Work out the finished part from the listing and answer in its coordinate system (mm). A direction names the side the tool comes from. Coordinates: 2 decimals unless noted, no trailing zeros. Loops run counter-clockwise (first coordinate to the right, second up) from the corner with the lowest first, then second, coordinate; pieces in that order, holes last.
```python
from build123d import *

# Parameters (mm, degrees)
SKETCH_1_W          = 109
SKETCH_1_H          = 63
EXTRUDE_1_DEPTH     = 5
CHAMFER_1_SIZE      = 3
SKETCH_2_W          = 75
SKETCH_2_H          = 45
EXTRUDE_2_DEPTH     = 20
SKETCH_3_W          = 70
SKETCH_3_H          = 27
CUT_EXTRUDE_1_DEPTH = 18
SKETCH_4_W          = 73
SKETCH_4_H          = 43
CUT_EXTRUDE_2_DEPTH = 15
SKETCH_5_R          = 2
EXTRUDE_3_DEPTH     = 10
FILLET_1_R          = 2


with BuildPart() as part:
    # 草图1 → 凸台-拉伸1 (new body)
    with BuildSketch(Plane.XY):
        Rectangle(SKETCH_1_W, SKETCH_1_H)
    extrude(amount=EXTRUDE_1_DEPTH)

    # 倒角1
    chamfer_1_edges = [part.edges().sort_by_distance(p)[0] for p in [
        (-54.5, 0, 5),
        (0, -31.5, 5),
        (54.5, 0, 5),
        (0, 31.5, 5),
    ]]
    chamfer(chamfer_1_edges, length=CHAMFER_1_SIZE)

    # 草图2 → 凸台-拉伸2 (add)
    with BuildSketch(Plane.XY.offset(5)):
        Rectangle(SKETCH_2_W, SKETCH_2_H)
    extrude(amount=-EXTRUDE_2_DEPTH)

    # 草图3 → 切除-拉伸1 (cut)
    with BuildSketch(Plane.XY.offset(5)):
        Rectangle(SKETCH_3_W, SKETCH_3_H)
    extrude(amount=-CUT_EXTRUDE_1_DEPTH, mode=Mode.SUBTRACT)

    # 草图4 → 切除-拉伸2 (cut)
    with BuildSketch(Plane.XY.offset(-13)):
        Rectangle(SKETCH_4_W, SKETCH_4_H)
    extrude(amount=CUT_EXTRUDE_2_DEPTH, mode=Mode.SUBTRACT)

    # 草图5 → 凸台-拉伸3 (add)
    with BuildSketch(Plane(origin=(0, 0, 0), x_dir=(-1, 0, 0), z_dir=(0, 0, -1))):
        with Locations((44, 19)):
            Circle(SKETCH_5_R)
        with Locations((44, -19)):
            Circle(SKETCH_5_R)
        with Locations((-44, -19)):
            Circle(SKETCH_5_R)
        with Locations((-44, 19)):
            Circle(SKETCH_5_R)
    extrude(amount=EXTRUDE_3_DEPTH)

    # 圆角1
    fillet_1_edges = [part.edges().sort_by_distance(p)[0] for p in [
        (37.5, 0, -15),
        (0, -22.5, -15),
        (-37.5, 0, -15),
        (0, 22.5, -15),
    ]]
    fillet(fillet_1_edges, radius=FILLET_1_R)


solid = part.part
```
1. Each of these flat-tipped pins is pushed along its axis until it touches: P1, Ø4.5, axis at x = -44.5, y = -19.5, coming from the -Z side; P2, Ø5, axis at y = -9, z = -12, coming from the +X side; P3, Ø8, axis at y = 4, z = -13, coming from the -X side; P4, Ø10, axis at x = -14, z = 2.5, coming from the -Y side. Where does it stop, or does it pass through?
2. Determine the mould class of faces 1 (the flat face through (36.5, 0, -6)), 2 (the cylindrical face through (36.93, 0.32, -14.4)), 3 (the flat face through (-1, -31.5, 1)), 4 (the flat face through (-53, -0.4, 3.5)) for opening direction X: released by +X, released by -X, zero draft, split by the parting line, or undercut.
3. A cutting plane is placed at D-D, the plane x = 44. Give the vertices of the cut face in (y, z).
4. A cutting plane is placed at B-B, the plane y = -19. Give the vertices of the cut face in (x, z), then the cut area to 3 significant figures.
5. Straight lines are drawn through the part: probe 1 along Y at (x, z) = (-12, -9.75); probe 2 along Z at (x, y) = (-2.5, -20.5); probe 3 along X at (y, z) = (-13, -11.75). For each, find the intervals that lie inside material, in ascending order.
6. A cutting plane is placed at A-A, the plane z = -6. Give the vertices of the cut face in (x, y), then the cut area to 3 significant figures.
7. For faces 5 (the flat face through (-37.5, 0, -6)), 6 (the flat face through (0, -13.5, 4)), 7 (the flat face through (-44, -19, -10)), 8 (the flat face through (-1, 22.5, -6)), 9 (the flat face through (-1, 21.5, -6)), determine the directions among +Z, -Z, +X, -X, +Y, -Y from which every point of the face is accessible in a straight line to the end or side of a thin tool.
8. A cutting plane is placed at C-C, the plane z = -11.5. Give the vertices of the cut face in (x, y).
Answers below:
1. P1: stops at z = -10
1. P2: stops at x = 37.5
1. P3: stops at x = -37.5
1. P4: stops at y = -31.5
2. face 1: undercut
2. face 2: released by +X
2. face 3: zero draft
2. face 4: released by -X
3. outline: (-31.5, 0) - (-21, 0) - (-21, -10) - (-17, -10) - (-17, 0) - (17, 0) - (17, -10) - (21, -10) - (21, 0) - (31.5, 0) - (31.5, 2) - (28.5, 5) - (-28.5, 5) - (-31.5, 2) - close
4. outline: (-54.5, 0) - (-46, 0) - (-46, -10) - (-42, -10) - (-42, 0) - (-37.5, 0) - (-37.5, -13) arc R2 ccw to (-35.5, -15) - (35.5, -15) arc R2 ccw to (37.5, -13) - (37.5, 0) - (42, 0) - (42, -10) - (46, -10) - (46, 0) - (54.5, 0) - (54.5, 2) - (51.5, 5) - (-51.5, 5) - (-54.5, 2) - close; hole (-36.5, -13) - (36.5, -13) - (36.5, 2) - (-36.5, 2) - close
4. area: 644 mm2
5. probe 1: y = -22.5 to -21.5, 21.5 to 22.5
5. probe 2: z = -15 to -13, 2 to 5
5. probe 3: x = -37.5 to -36.5, 36.5 to 37.5
6. outline: circle Ø4 at (-44, -19); circle Ø4 at (-44, 19); (-37.5, -22.5) - (37.5, -22.5) - (37.5, 22.5) - (-37.5, 22.5) - close; circle Ø4 at (44, -19); circle Ø4 at (44, 19); hole (-36.5, -21.5) - (36.5, -21.5) - (36.5, 21.5) - (-36.5, 21.5) - close
6. area: 286 mm2
7. face 5: -Z, +Y, -Y
7. face 6: +Z
7. face 7: -Z, -X, +Y, -Y
7. face 8: -Z, +X, -X, +Y
7. face 9: none
8. outline: (-37.5, -22.5) - (37.5, -22.5) - (37.5, 22.5) - (-37.5, 22.5) - close; hole (-36.5, -21.5) - (36.5, -21.5) - (36.5, 21.5) - (-36.5, 21.5) - close
